Here's how the part is built. I have some questions about the finished solid (model axes, mm). Give positions to 0.01 mm unless a question says otherwise; leave off trailing zeros. Loops run counter-clockwise (first coordinate to the right, second up) from the corner with the lowest first, then second, coordinate; pieces in that order, holes last. Notation, with made-up numbers: (27, -18) - (56, -18) arc R7 cw to (56, -9) - close; hole circle Ø2 at (3, 44.25). An arc over 180 degrees is marked (long way). Use one line per item in the form item = value.
from build123d import *

# Parameters (mm, degrees)
SKETCH3_R           = 105
SKETCH3_R_2         = 18
SKETCH3_R_3         = 9
BOSS_EXTRUDE2_DEPTH = 10


with BuildPart() as part:
    # Sketch3 → Boss-Extrude2 (new body)
    with BuildSketch(Plane(origin=(0, 0, 0), x_dir=(1, 0, 0), z_dir=(0, 1, 0))):
        with Locations(Location((0, 0, 0), (0, 0, 270))):
            Circle(SKETCH3_R)
        with Locations(Location((-21.213203436, -21.213203436, 0), (0, 0, 270))):
            Circle(SKETCH3_R_2, mode=Mode.SUBTRACT)
        with Locations(Location((21.213203436, -21.213203436, 0), (0, 0, 270))):
            Circle(SKETCH3_R_2, mode=Mode.SUBTRACT)
        with Locations(Location((0, 30, 0), (0, 0, 270))):
            Circle(SKETCH3_R_2, mode=Mode.SUBTRACT)
        with Locations(Location((87.5, 0, 0), (0, 0, 270))):
            Circle(SKETCH3_R_3, mode=Mode.SUBTRACT)
        with Locations(Location((61.871843354, -61.871843354, 0), (0, 0, 270))):
            Circle(SKETCH3_R_3, mode=Mode.SUBTRACT)
        with Locations(Location((0, -87.5, 0), (0, 0, 270))):
            Circle(SKETCH3_R_3, mode=Mode.SUBTRACT)
        with Locations(Location((-61.871843354, -61.871843354, 0), (0, 0, 270))):
            Circle(SKETCH3_R_3, mode=Mode.SUBTRACT)
        with Locations(Location((-87.5, 0, 0), (0, 0, 270))):
            Circle(SKETCH3_R_3, mode=Mode.SUBTRACT)
        with Locations(Location((-61.871843354, 61.871843354, 0), (0, 0, 270))):
            Circle(SKETCH3_R_3, mode=Mode.SUBTRACT)
        with Locations(Location((61.871843354, 61.871843354, 0), (0, 0, 270))):
            Circle(SKETCH3_R_3, mode=Mode.SUBTRACT)
        with Locations(Location((0, 87.5, 0), (0, 0, 270))):
            Circle(SKETCH3_R_3, mode=Mode.SUBTRACT)
        with BuildLine():
            ThreePointArc((29.933258413, 23.222683604), (24.521297412, 10.157053955), (37.586927061, 4.745092953))
            Line((37.586927061, 4.745092953), (51.445120048, 10.485344439))
            ThreePointArc((51.445120048, 10.485344439), (56.85708105, 23.550974088), (43.791451401, 28.962935089))
            Line((43.791451401, 28.962935089), (29.933258413, 23.222683604))
        make_face(mode=Mode.SUBTRACT)
    extrude(amount=BOSS_EXTRUDE2_DEPTH)


solid = part.part
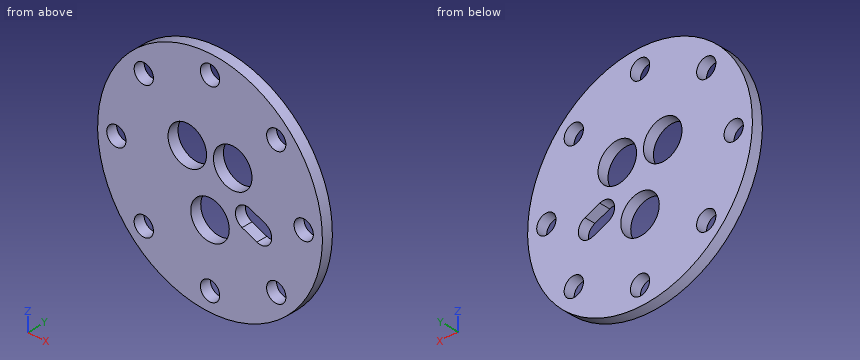
(1) For P1, Ø5, axis at y = 6.5, z = -71, coming from the +X side; P2, Ø16, axis at x = 61.87, z = -61.87, coming from the +Y side; P3, Ø1.5, axis at x = -10, y = 4.5, coming from the +Z side; P4, Ø2, axis at x = 69.5, y = 9, coming from the +Z side, each with a flat end and sliding along its axis, tell me the tip position at first contact or that it passes through.
Geometry says:
P1 = 79.58
P2 = through
P3 = 104.59
P4 = 79.58
(2) If we section it at C-C (z = -87.5): List the corners of the cut face in (x, y) for me, plus the area to 3 significant figures.
Geometry says:
outline = (-58.04, 0) - (-9, 0) - (-9, 10) - (-58.04, 10) - close; (9, 0) - (58.04, 0) - (58.04, 10) - (9, 10) - close
area = 981 mm²
(3) If we section it at D-D (y = 8): Give the number of separate pieces and of enclosed holes in the cut face, plus the area to 3 significant figures.
Geometry says:
separate_pieces = 1
enclosed_holes = 12
area = 28,900 mm²
(4) If we section it at A-A (x = 0): List the corners of the cut face in (y, z) for me, plus the area to 3 significant figures.
Geometry says:
outline = (0, -105) - (10, -105) - (10, -96.5) - (0, -96.5) - close; (0, -78.5) - (10, -78.5) - (10, -48) - (0, -48) - close; (0, -12) - (10, -12) - (10, 78.5) - (0, 78.5) - close; (0, 96.5) - (10, 96.5) - (10, 105) - (0, 105) - close
area = 1,380 mm²
(5) If we section it at B-B (z = 0): List the corners of the cut face in (x, y) for me.
Geometry says:
outline = (-105, 0) - (-96.5, 0) - (-96.5, 10) - (-105, 10) - close; (-78.5, 0) - (78.5, 0) - (78.5, 10) - (-78.5, 10) - close; (96.5, 0) - (105, 0) - (105, 10) - (96.5, 10) - close
(6) If I drill on probe 1 along Z at (x, y) = (16, 7); probe 2 along X at (y, z) = (8.25, 65); probe 3 along X at (y, z) = (2, 6), over which ranges is the centre line in solid material (lowest first)?
Geometry says:
probe_1 = -103.77 to -38.25, -21.75 to 3.98, 38.44 to 103.77
probe_2 = -82.46 to -70.31, -53.43 to 53.43, 70.31 to 82.46
probe_3 = -104.83 to -94.21, -80.79 to -30.83, -11.59 to 11.59, 30.83 to 80.79, 94.21 to 104.83
